Check sheet for the modelled part. Datum: model origin and axes. Units: mm. A direction names the side the tool comes from. Coordinates: 2 decimals unless noted, no trailing zeros. Write each loop counter-clockwise with the first axis right and the second up, starting at its lowest first coordinate (ties: lowest second). Pieces come first, ordered by that corner, then holes. Notation, with made-up numbers: M 20.25,70 L 55.25,70 A7 ccw 55.25,83 Z; hole C -5,-38.5 d8. An arc over 180 degrees is marked long. Answer as CSV lines item,"result".
from build123d import *

# Parameters (mm, degrees)
PRISM002_DEPTH         = 10
PRISM002_ROLL_ANGLE    = -90
CYLINDER051_R          = 3
CYLINDER051_DEPTH      = 32
CYLINDER051_ROLL_ANGLE = -90
CYLINDER052_R          = 3
CYLINDER052_DEPTH      = 32
CYLINDER052_ROLL_ANGLE = -90
BOX040_W               = 20
BOX040_H               = 16
BOX040_DEPTH           = 28
CYLINDER053_R          = 1.75
CYLINDER053_DEPTH      = 32
CYLINDER053_ROLL_ANGLE = -90
CYLINDER054_R          = 1.75
CYLINDER054_DEPTH      = 32
CYLINDER054_ROLL_ANGLE = -90
PRISM001_DEPTH         = 10
PRISM001_ROLL_ANGLE    = -90


with BuildPart() as prisma002:
    # Prism002 → Prism002 (new body)
    with BuildSketch(Plane.XY):
        Polygon((3.3, 0), (1.65, 2.857884), (-1.65, 2.857884), (-3.3, 0), (-1.65, -2.857884), (1.65, -2.857884), align=None)
    extrude(amount=PRISM002_DEPTH)


with BuildPart() as prisma002_1:
    # Prism002 roll: moved
    add(prisma002.part.rotate(Axis((0, 0, 0), (1, 0, 0)), PRISM002_ROLL_ANGLE))


with BuildPart() as prisma002_2:
    # Prism002 placement: moved
    add(prisma002_1.part.moved(Location((8, 85, 84))))


with BuildPart() as cilindro017:
    # Cylinder051 → Cylinder051 (new body)
    with BuildSketch(Plane.XY):
        Circle(CYLINDER051_R)
    extrude(amount=CYLINDER051_DEPTH)


with BuildPart() as cilindro017_1:
    # Cylinder051 roll: moved
    add(cilindro017.part.rotate(Axis((0, 0, 0), (1, 0, 0)), CYLINDER051_ROLL_ANGLE))


with BuildPart() as cilindro017_2:
    # Cylinder051 placement: moved
    add(cilindro017_1.part.moved(Location((18, 116, 84))))


with BuildPart() as cilindro018:
    # Cylinder052 → Cylinder052 (new body)
    with BuildSketch(Plane.XY):
        Circle(CYLINDER052_R)
    extrude(amount=CYLINDER052_DEPTH)


with BuildPart() as cilindro018_1:
    # Cylinder052 roll: moved
    add(cilindro018.part.rotate(Axis((0, 0, 0), (1, 0, 0)), CYLINDER052_ROLL_ANGLE))


with BuildPart() as cilindro018_2:
    # Cylinder052 placement: moved
    add(cilindro018_1.part.moved(Location((8, 116, 84))))


with BuildPart() as cubo005:
    # Box040 → Box040 (new body)
    with BuildSketch(Plane(origin=(3.5, 97.5, 79.5), x_dir=(1, 0, 0), z_dir=(0, 0, 1))):
        with Locations((10, 8)):
            Rectangle(BOX040_W, BOX040_H)
    extrude(amount=BOX040_DEPTH)


with BuildPart() as cilindro013:
    # Cylinder053 → Cylinder053 (new body)
    with BuildSketch(Plane.XY):
        Circle(CYLINDER053_R)
    extrude(amount=CYLINDER053_DEPTH)


with BuildPart() as cilindro013_1:
    # Cylinder053 roll: moved
    add(cilindro013.part.rotate(Axis((0, 0, 0), (1, 0, 0)), CYLINDER053_ROLL_ANGLE))


with BuildPart() as cilindro013_2:
    # Cylinder053 placement: moved
    add(cilindro013_1.part.moved(Location((18, 90, 84))))


with BuildPart() as cilindro012:
    # Cylinder054 → Cylinder054 (new body)
    with BuildSketch(Plane.XY):
        Circle(CYLINDER054_R)
    extrude(amount=CYLINDER054_DEPTH)


with BuildPart() as cilindro012_1:
    # Cylinder054 roll: moved
    add(cilindro012.part.rotate(Axis((0, 0, 0), (1, 0, 0)), CYLINDER054_ROLL_ANGLE))


with BuildPart() as cilindro012_2:
    # Cylinder054 placement: moved
    add(cilindro012_1.part.moved(Location((8, 90, 84))))


with BuildPart() as arm_positive_cut:
    # Prism001 → Prism001 (new body)
    with BuildSketch(Plane.XY):
        Polygon((3.3, 0), (1.65, 2.857884), (-1.65, 2.857884), (-3.3, 0), (-1.65, -2.857884), (1.65, -2.857884), align=None)
    extrude(amount=PRISM001_DEPTH)


with BuildPart() as arm_positive_cut_1:
    # Prism001 roll: moved
    add(arm_positive_cut.part.rotate(Axis((0, 0, 0), (1, 0, 0)), PRISM001_ROLL_ANGLE))


with BuildPart() as arm_positive_cut_2:
    # Prism001 placement: moved
    add(arm_positive_cut_1.part.moved(Location((18, 85, 84))))

    # Fusion036: union Prisma002, Cilindro017, Cilindro018, Cubo005, Cilindro013, Cilindro012
    add(prisma002_2.part)
    add(cilindro017_2.part)
    add(cilindro018_2.part)
    add(cubo005.part)
    add(cilindro013_2.part)
    add(cilindro012_2.part)


solid = arm_positive_cut_2.part
1) Section check C-C, the plane z = 96.25. Record the boundary of the cut face in (x, y), plus the area to 3 significant figures.
Answer key:
outline,"M 3.5,97.5 L 23.5,97.5 L 23.5,113.5 L 3.5,113.5 Z"
area,"320 mm2"
2) Depth check by flat-ended pin: P1, Ø4, axis at x = 16.5, z = 93.5, coming from the -Y side; P2, Ø1, axis at y = 128, z = 84.5, coming from the -X side; P3, Ø2.5, axis at x = 8.5, y = 90, coming from the +Z side. Enter the tip coordinate at first touch or a pass-through.
Answer key:
P1,"stops at y = 97.5"
P2,"stops at x = 5"
P3,"stops at z = 86.86"
3) Tool access check on faces 1 (the face through (8.81, 114.73, 85.55)), 2 (the face through (5.513, 89.93, 85.409)), 3 (the face through (5.537, 89.93, 82.551)). Record the directions out of +Z, -Z, +X, -X, +Y, -Y that give a thin tool (end or side, any length) a straight path to the whole face; none if there is none.
Answer key:
face 1,"none"
face 2,"+Z, -X, -Y"
face 3,"-Z, -X, -Y"
4) Section check A-A, the plane x = 18. Record the boundary of the cut face in (y, z).
Answer key:
outline,"M 85,81.14 L 95,81.14 L 95,82.25 L 97.5,82.25 L 97.5,79.5 L 113.5,79.5 L 113.5,82.25 L 116,82.25 L 116,81 L 148,81 L 148,87 L 116,87 L 116,85.75 L 113.5,85.75 L 113.5,107.5 L 97.5,107.5 L 97.5,85.75 L 95,85.75 L 95,86.86 L 85,86.86 Z"
5) Thickness scan on line 1 along Y through (x, z) = (9.75, 83.5); line 2 along X through (y, z) = (124.5, 86.5); line 3 along Y through (x, z) = (9.5, 100.5). Record the ranges inside material, lowest first.
Answer key:
line 1,"y = 85 to 95, 97.5 to 113.5, 116 to 148"
line 2,"x = 6.34 to 9.66, 16.34 to 19.66"
line 3,"y = 97.5 to 113.5"
6) Mould release check, pull along Y, two halves, no side actions. Record for faces 4 (the face through (18, 85, 84)), 5 (the face through (20, 116, 84)), 6 (the face through (17.35, 131.78, 86.93)): pulls with the +Y half, pulls with the -Y half, needs draft (parallel to the pull), parting line crosses it, or undercut.
Answer key:
face 4,"pulls with the -Y half"
face 5,"undercut"
face 6,"needs draft"
7) Section check B-B, the plane y = 123. Record the boundary of the cut face in (x, z), plus the area to 3 significant figures.
Answer key:
outline,"C 8,84 d6; C 18,84 d6"
area,"56.5 mm2"
